Here's the drawing with two shaded views (mm, measured from the low corner). I have some questions. Round coordinates to 2 decimals unless told otherwise and drop trailing zeros. Loops run counter-clockwise (first coordinate to the right, second up) from the corner with the lowest first, then second, coordinate; pieces in that order, holes last. Notation, with made-up numbers: M -15,31 L 27,31 A27 ccw 27,56 Z; hole C -10,-29 d2. An arc over 180 degrees is marked long. One line per item, written item: value. Start each with the question number.
Q1. Imagine slicing it at D-D (y = 67.55). Please give me the cut outline in (x, z) (3 decimals), then the cut area to 3 significant figures.
Q2. Thinking about a two-plate mould opening in Z: for the marked faces 1 and 2, which applies, released by +Z, released by -Z, zero draft, split by the parting line, or undercut?
Q3. Imagine slicing it at A-A (y = 20.5). Please give me the cut outline in (x, z).
Q4. Please list where these lines run through material, in increasing order: line 1 along Z through (x, y) = (60, 27); line 2 along Z through (x, y) = (19.65, 9.25) (3 decimals); line 3 along X through (y, z) = (111, 75).
Q5. I'm going to push flat-ended pins straight in: pin 1 Ø8 at (y, z) = (59, 177) entering from +X; pin 2 Ø5 at (x, z) = (48.758, 110.725) entering from -Y; pin 3 Ø3 at (x, z) = (182.5, 4) entering from -Y; pin 4 Ø3 at (x, y) = (3.5, 64.5) entering from +Z. Where does each tip first touch, or does it pass through?
Q6. Imagine slicing it at C-C (z = 132.5). Please give me the cut outline in (x, y), then the cut area to 3 significant figures.
Q7. Imagine slicing it at B-B (x = 26). Please give me the cut outline in (y, z).
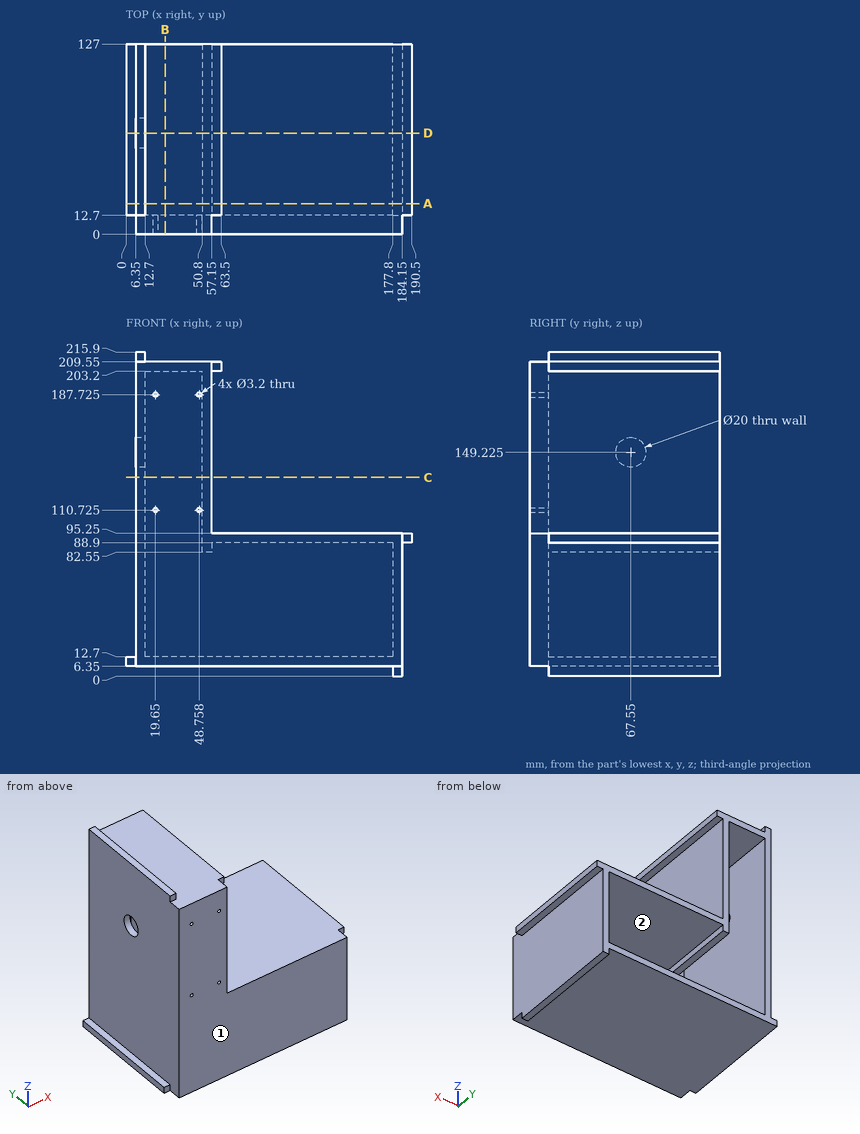
Report:
1. outline: M 0,6.35 L 177.8,6.35 L 177.8,0 L 184.15,0 L 184.15,88.9 L 190.5,88.9 L 190.5,95.25 L 57.15,95.25 L 57.15,203.2 L 63.5,203.2 L 63.5,209.55 L 12.7,209.55 L 12.7,215.9 L 6.35,215.9 L 6.35,159.225 L 12.7,159.225 L 12.7,203.2 L 50.8,203.2 L 50.8,82.55 L 57.15,82.55 L 57.15,88.9 L 177.8,88.9 L 177.8,12.7 L 12.7,12.7 L 12.7,139.225 L 6.35,139.225 L 6.35,12.7 L 0,12.7 Z
1. area: 4,790 mm²
2. face 1: zero draft
2. face 2: undercut
3. outline: M 0,6.35 L 177.8,6.35 L 177.8,0 L 184.15,0 L 184.15,88.9 L 190.5,88.9 L 190.5,95.25 L 57.15,95.25 L 57.15,203.2 L 63.5,203.2 L 63.5,209.55 L 12.7,209.55 L 12.7,215.9 L 6.35,215.9 L 6.35,12.7 L 0,12.7 Z; hole M 12.7,12.7 L 177.8,12.7 L 177.8,88.9 L 57.15,88.9 L 57.15,82.55 L 50.8,82.55 L 50.8,203.2 L 12.7,203.2 Z
4. line 1: z = 6.35 to 12.7, 88.9 to 95.25, 203.2 to 209.55
4. line 2: z = 6.35 to 109.125, 112.325 to 186.125, 189.325 to 209.55
4. line 3: x = 6.35 to 12.7, 177.8 to 184.15
5. pin 1: stops at x = 57.15
5. pin 2: stops at y = 0
5. pin 3: stops at y = 12.7
5. pin 4: stops at z = 12.7
6. outline: M 6.35,0 L 57.15,0 L 57.15,127 L 50.8,127 L 50.8,12.7 L 12.7,12.7 L 12.7,127 L 6.35,127 Z
6. area: 2,100 mm²
7. outline: M 0,6.35 L 127,6.35 L 127,12.7 L 12.7,12.7 L 12.7,203.2 L 127,203.2 L 127,209.55 L 0,209.55 Z
